Check sheet for the modelled part. Datum: model origin and axes. Units: mm. Give positions to 0.01 mm unless a question says otherwise; leave off trailing zeros. Loops run counter-clockwise (first coordinate to the right, second up) from the corner with the lowest first, then second, coordinate; pieces in that order, holes last. Notation, with made-up numbers: M -27,22 L 18,22 A9 ccw 18,32 Z; hole C 13,-16 d11. An arc over 180 degrees is marked long. Write each question's results on one line, items separated by ' | '. Start each with the question number.
1. Sectioned sample at A-A on z = 60.5. Record the cut outline in (x, y), and give its area (3 significant figures).
2. Sectioned sample at B-B on x = 130.5. Give the number of separate pieces and of enclosed holes in the cut face, and give its area (3 significant figures).
3. Material ranges on line 1 along X through (y, z) = (3.95, 25.5); line 2 along X through (y, z) = (2.55, 103.5); line 3 along Z through (x, y) = (17.5, 1.35), recorded low to high.
4. Draft check along Z on faces 1 (the flat face through (0, 2, 97)), 2 (the cylindrical face through (107.305, 2.465, 138.026)). Enter one of: pulls with the +Z half, pulls with the -Z half, needs draft (parallel to the pull), parting line crosses it, or undercut.
5. Sectioned sample at C-C on x = 79. Record the cut outline in (y, z).
6. Sectioned sample at D-D on z = 157. Record the cut outline in (x, y), and give its area (3 significant figures).
7. Go/stop test with a flat-tipped pin: pin 1 (0.7 mm diameter, centred on x = 48, z = -1.5, fed in from +Y). Record where the tip stops, or that it passes through.
```python
from build123d import *

# Parameters (mm, degrees)
SKETCH1_W           = 156
SKETCH1_H           = 191
SKETCH1_R           = 14
BOSS_EXTRUDE1_DEPTH = 5
SKETCH2_W           = 156
SKETCH2_H           = 2
BOSS_EXTRUDE2_DEPTH = 2.45
SKETCH3_W           = 156
SKETCH3_H           = 2
BOSS_EXTRUDE3_DEPTH = 2.45


with BuildPart() as part:
    # Sketch1 → Boss-Extrude1 (new body)
    with BuildSketch(Plane(origin=(0, 0, 0), x_dir=(1, 0, 0), z_dir=(0, 1, 0))):
        with Locations((78, -95.5)):
            Rectangle(SKETCH1_W, SKETCH1_H)
        with Locations(Location((25.5, -165.5, 0), (0, 0, 270))):
            Circle(SKETCH1_R, mode=Mode.SUBTRACT)
        with Locations(Location((60.5, -165.5, 0), (0, 0, 270))):
            Circle(SKETCH1_R, mode=Mode.SUBTRACT)
        with Locations(Location((95.5, -165.5, 0), (0, 0, 270))):
            Circle(SKETCH1_R, mode=Mode.SUBTRACT)
        with Locations(Location((130.5, -165.5, 0), (0, 0, 270))):
            Circle(SKETCH1_R, mode=Mode.SUBTRACT)
        with Locations(Location((60.5, -130.5, 0), (0, 0, 270))):
            Circle(SKETCH1_R, mode=Mode.SUBTRACT)
        with Locations(Location((95.5, -130.5, 0), (0, 0, 270))):
            Circle(SKETCH1_R, mode=Mode.SUBTRACT)
        with Locations(Location((130.5, -130.5, 0), (0, 0, 270))):
            Circle(SKETCH1_R, mode=Mode.SUBTRACT)
        with Locations(Location((60.5, -95.5, 0), (0, 0, 270))):
            Circle(SKETCH1_R, mode=Mode.SUBTRACT)
        with Locations(Location((95.5, -95.5, 0), (0, 0, 270))):
            Circle(SKETCH1_R, mode=Mode.SUBTRACT)
        with Locations(Location((130.5, -95.5, 0), (0, 0, 270))):
            Circle(SKETCH1_R, mode=Mode.SUBTRACT)
        with Locations(Location((60.5, -60.5, 0), (0, 0, 270))):
            Circle(SKETCH1_R, mode=Mode.SUBTRACT)
        with Locations(Location((95.5, -60.5, 0), (0, 0, 270))):
            Circle(SKETCH1_R, mode=Mode.SUBTRACT)
        with Locations(Location((130.5, -60.5, 0), (0, 0, 270))):
            Circle(SKETCH1_R, mode=Mode.SUBTRACT)
        with Locations(Location((60.5, -25.5, 0), (0, 0, 270))):
            Circle(SKETCH1_R, mode=Mode.SUBTRACT)
        with Locations(Location((95.5, -25.5, 0), (0, 0, 270))):
            Circle(SKETCH1_R, mode=Mode.SUBTRACT)
        with Locations(Location((130.5, -25.5, 0), (0, 0, 270))):
            Circle(SKETCH1_R, mode=Mode.SUBTRACT)
        with Locations(Location((25.5, -130.5, 0), (0, 0, 270))):
            Circle(SKETCH1_R, mode=Mode.SUBTRACT)
        with Locations(Location((25.5, -95.5, 0), (0, 0, 270))):
            Circle(SKETCH1_R, mode=Mode.SUBTRACT)
        with Locations(Location((25.5, -60.5, 0), (0, 0, 270))):
            Circle(SKETCH1_R, mode=Mode.SUBTRACT)
        with Locations(Location((25.5, -25.5, 0), (0, 0, 270))):
            Circle(SKETCH1_R, mode=Mode.SUBTRACT)
    extrude(amount=BOSS_EXTRUDE1_DEPTH)

    # Sketch2 → Boss-Extrude2 (add)
    with BuildSketch(Plane.XY.offset(191)):
        with Locations((78, 2)):
            Rectangle(SKETCH2_W, SKETCH2_H)
    extrude(amount=BOSS_EXTRUDE2_DEPTH)

    # Sketch3 → Boss-Extrude3 (add)
    with BuildSketch(Plane(origin=(0, 0, 0), x_dir=(-1, 0, 0), z_dir=(0, 0, -1))):
        with Locations((-78, 2)):
            Rectangle(SKETCH3_W, SKETCH3_H)
    extrude(amount=BOSS_EXTRUDE3_DEPTH)


solid = part.part
```
Output values:
1) outline: M 0,0 L 11.5,0 L 11.5,5 L 0,5 Z; M 39.5,0 L 46.5,0 L 46.5,5 L 39.5,5 Z; M 74.5,0 L 81.5,0 L 81.5,5 L 74.5,5 Z; M 109.5,0 L 116.5,0 L 116.5,5 L 109.5,5 Z; M 144.5,0 L 156,0 L 156,5 L 144.5,5 Z | area: 220 mm2
2) separate pieces: 6 | enclosed holes: 0 | area: 265 mm2
3) line 1: 0 to 11.5, 39.5 to 46.5, 74.5 to 81.5, 109.5 to 116.5, 144.5 to 156 | line 2: 0 to 14.01, 36.99 to 49.01, 71.99 to 84.01, 106.99 to 119.01, 141.99 to 156 | line 3: -2.45 to 14.01, 36.99 to 49.01, 71.99 to 84.01, 106.99 to 119.01, 141.99 to 154.01, 176.99 to 193.45
4) face 1: needs draft | face 2: undercut
5) outline: M 0,0 L 1,0 L 1,-2.45 L 3,-2.45 L 3,0 L 5,0 L 5,191 L 3,191 L 3,193.45 L 1,193.45 L 1,191 L 0,191 Z
6) outline: M 0,0 L 14.38,0 L 14.38,5 L 0,5 Z; M 36.62,0 L 49.38,0 L 49.38,5 L 36.62,5 Z; M 71.62,0 L 84.38,0 L 84.38,5 L 71.62,5 Z; M 106.62,0 L 119.38,0 L 119.38,5 L 106.62,5 Z; M 141.62,0 L 156,0 L 156,5 L 141.62,5 Z | area: 335 mm2
7) pin 1: y = 3
